```python
from build123d import *

# Parameters (mm, degrees)
F0_R     = 38.1
F1_DEPTH = 5.08


with BuildPart() as f1:
    # F0 (on Top) → F1 (new body)
    with BuildSketch(Plane.XY):
        Circle(F0_R)
        with BuildLine():
            ThreePointArc((21.9970452561, 12.7), (24.5345159877, 6.5740037456), (25.4, 0))
            ThreePointArc((25.4, 0), (24.5345159877, -6.5740037456), (21.9970452561, -12.7))
            ThreePointArc((21.9970452561, -12.7), (17.9605122421, -17.9605122421), (12.7, -21.9970452561))
            ThreePointArc((12.7, -21.9970452561), (6.5740037456, -24.5345159877), (0, -25.4))
            ThreePointArc((0, -25.4), (-6.5740037456, -24.5345159877), (-12.7, -21.9970452561))
            ThreePointArc((-12.7, -21.9970452561), (-17.9605122421, -17.9605122421), (-21.9970452561, -12.7))
            ThreePointArc((-21.9970452561, -12.7), (-24.5345159877, -6.5740037456), (-25.4, 0))
            ThreePointArc((-25.4, 0), (-24.5345159877, 6.5740037456), (-21.9970452561, 12.7))
            ThreePointArc((-21.9970452561, 12.7), (-17.9605122421, 17.9605122421), (-12.7, 21.9970452561))
            ThreePointArc((-12.7, 21.9970452561), (-6.5740037456, 24.5345159877), (0, 25.4))
            ThreePointArc((0, 25.4), (6.5740037456, 24.5345159877), (12.7, 21.9970452561))
            ThreePointArc((12.7, 21.9970452561), (17.9605122421, 17.9605122421), (21.9970452561, 12.7))
        make_face(mode=Mode.SUBTRACT)
        with BuildLine():
            Line((-8.248891971, -4.7625), (0, 0))
            Line((0, 0), (-9.525, 0))
            ThreePointArc((-9.525, 0), (-9.2004434954, -2.4652514046), (-8.248891971, -4.7625))
        make_face()
        with BuildLine():
            Line((-4.7625, -8.248891971), (0, 0))
            Line((0, 0), (-8.248891971, -4.7625))
            ThreePointArc((-8.248891971, -4.7625), (-6.7351920908, -6.7351920908), (-4.7625, -8.248891971))
        make_face()
        with BuildLine():
            Line((0, -9.525), (0, 0))
            Line((0, 0), (-4.7625, -8.248891971))
            ThreePointArc((-4.7625, -8.248891971), (-2.4652514046, -9.2004434954), (0, -9.525))
        make_face()
        with BuildLine():
            Line((4.7625, -8.248891971), (0, 0))
            Line((0, 0), (0, -9.525))
            ThreePointArc((0, -9.525), (2.4652514046, -9.2004434954), (4.7625, -8.248891971))
        make_face()
        with BuildLine():
            ThreePointArc((4.7625, -8.248891971), (6.7351920908, -6.7351920908), (8.248891971, -4.7625))
            Line((8.248891971, -4.7625), (0, 0))
            Line((0, 0), (4.7625, -8.248891971))
        make_face()
        with BuildLine():
            ThreePointArc((8.248891971, -4.7625), (9.2004434954, -2.4652514046), (9.525, 0))
            Line((9.525, 0), (0, 0))
            Line((0, 0), (8.248891971, -4.7625))
        make_face()
        with BuildLine():
            Line((0, 0), (9.525, 0))
            ThreePointArc((9.525, 0), (9.2004434954, 2.4652514046), (8.248891971, 4.7625))
            Line((8.248891971, 4.7625), (0, 0))
        make_face()
        with BuildLine():
            Line((0, 0), (8.248891971, 4.7625))
            ThreePointArc((8.248891971, 4.7625), (6.7351920908, 6.7351920908), (4.7625, 8.248891971))
            Line((4.7625, 8.248891971), (0, 0))
        make_face()
        with BuildLine():
            Line((0, 9.525), (0, 0))
            Line((0, 0), (4.7625, 8.248891971))
            ThreePointArc((4.7625, 8.248891971), (2.4652514046, 9.2004434954), (0, 9.525))
        make_face()
        with BuildLine():
            Line((-4.7625, 8.248891971), (0, 0))
            Line((0, 0), (0, 9.525))
            ThreePointArc((0, 9.525), (-2.4652514046, 9.2004434954), (-4.7625, 8.248891971))
        make_face()
        with BuildLine():
            Line((-8.248891971, 4.7625), (0, 0))
            Line((0, 0), (-4.7625, 8.248891971))
            ThreePointArc((-4.7625, 8.248891971), (-6.7351920908, 6.7351920908), (-8.248891971, 4.7625))
        make_face()
        with BuildLine():
            Line((-9.525, 0), (0, 0))
            Line((0, 0), (-8.248891971, 4.7625))
            ThreePointArc((-8.248891971, 4.7625), (-9.2004434954, 2.4652514046), (-9.525, 0))
        make_face()
        with BuildLine():
            ThreePointArc((-9.525, 0), (-9.2004434954, 2.4652514046), (-8.248891971, 4.7625))
            Line((-8.248891971, 4.7625), (-21.9970452561, 12.7))
            ThreePointArc((-21.9970452561, 12.7), (-24.5345159877, 6.5740037456), (-25.4, 0))
            Line((-25.4, 0), (-9.525, 0))
        make_face()
        with BuildLine():
            Line((0, 9.525), (0, 25.4))
            ThreePointArc((0, 25.4), (-6.5740037456, 24.5345159877), (-12.7, 21.9970452561))
            Line((-12.7, 21.9970452561), (-4.7625, 8.248891971))
            ThreePointArc((-4.7625, 8.248891971), (-2.4652514046, 9.2004434954), (0, 9.525))
        make_face()
        with BuildLine():
            Line((8.248891971, 4.7625), (21.9970452561, 12.7))
            ThreePointArc((21.9970452561, 12.7), (17.9605122421, 17.9605122421), (12.7, 21.9970452561))
            Line((12.7, 21.9970452561), (4.7625, 8.248891971))
            ThreePointArc((4.7625, 8.248891971), (6.7351920908, 6.7351920908), (8.248891971, 4.7625))
        make_face()
        with BuildLine():
            ThreePointArc((21.9970452561, -12.7), (24.5345159877, -6.5740037456), (25.4, 0))
            Line((25.4, 0), (9.525, 0))
            ThreePointArc((9.525, 0), (9.2004434954, -2.4652514046), (8.248891971, -4.7625))
            Line((8.248891971, -4.7625), (21.9970452561, -12.7))
        make_face()
        with BuildLine():
            ThreePointArc((0, -25.4), (6.5740037456, -24.5345159877), (12.7, -21.9970452561))
            Line((12.7, -21.9970452561), (4.7625, -8.248891971))
            ThreePointArc((4.7625, -8.248891971), (2.4652514046, -9.2004434954), (0, -9.525))
            Line((0, -9.525), (0, -25.4))
        make_face()
        with BuildLine():
            ThreePointArc((-4.7625, -8.248891971), (-6.7351920908, -6.7351920908), (-8.248891971, -4.7625))
            Line((-8.248891971, -4.7625), (-21.9970452561, -12.7))
            ThreePointArc((-21.9970452561, -12.7), (-17.9605122421, -17.9605122421), (-12.7, -21.9970452561))
            Line((-12.7, -21.9970452561), (-4.7625, -8.248891971))
        make_face()
    extrude(amount=F1_DEPTH)


solid = f1.part
```
Work out the finished part from the listing and answer in its coordinate system (mm). A direction names the side the tool comes from. Give positions to 0.01 mm unless a question says otherwise; leave off trailing zeros. Loops run counter-clockwise (first coordinate to the right, second up) from the corner with the lowest first, then second, coordinate; pieces in that order, holes last. Notation, with made-up numbers: (86, 3) - (93, 3) arc R28 ccw to (93, 32) - close; hole circle Ø8 at (-21.5, -32.5). An arc over 180 degrees is marked (long way). One line per question, with ' | ' between items.
(1) The part is cut by section B-B (x = 20.5). Write down the section's boundary in (y, z).
Recorded:
outline: (-32.11, 0) - (-15, 0) - (-15, 5.08) - (-32.11, 5.08) - close; (-11.84, 0) - (0, 0) - (0, 5.08) - (-11.84, 5.08) - close; (11.84, 0) - (32.11, 0) - (32.11, 5.08) - (11.84, 5.08) - close
(2) The part is cut by section C-C (z = 3.25). Count the separate pieces of the cut face and the enclosed holes in it, then the cut area to 3 significant figures.
Recorded:
separate pieces: 1 | enclosed holes: 6 | area: 3,690 mm²
(3) A tool of negligible diameter and unlimited length cuts with its end or side. For faces 1 (the face through (-1, 1, 5.08)), 2 (the face through (-15.027, -8.676, 2.504)), from which of +Z, -Z, +X, -X, +Y, -Y can it reach the whole face along a straight path? Write none if from no direction.
Recorded:
face 1: +Z, +X, -X, +Y, -Y | face 2: +Z, -Z
(4) Each of these flat-tipped pins is pushed along its axis until it touches: pin 1 Ø2 at (x, z) = (6, 2.5) entering from -Y; pin 2 Ø1 at (x, z) = (-8.5, 0.5) entering from -Y; pin 3 Ø3 at (x, z) = (-22, 1) entering from -Y. Where does it stop, or does it pass through?
Recorded:
pin 1: stops at y = -37.77 | pin 2: stops at y = -37.25 | pin 3: stops at y = -32.11
(5) The mould has two halves that part along Y. Classify faces 3 (the face through (-1, 1, 0)), 4 (the face through (-24.5, -6.7, 2.5)): +Y half, -Y half, draft (parallel to the pull), parting line (faces both ways), or undercut.
Recorded:
face 3: draft | face 4: undercut
(6) The part is cut by section D-D (y = -15). Write down the section's boundary in (x, z), then the cut area to 3 significant figures.
Recorded:
outline: (-35.02, 0) - (-8.66, 0) - (-8.66, 5.08) - (-35.02, 5.08) - close; (0, 0) - (8.66, 0) - (8.66, 5.08) - (0, 5.08) - close; (20.5, 0) - (35.02, 0) - (35.02, 5.08) - (20.5, 5.08) - close | area: 252 mm²
(7) Straight lines are drawn through the part: probe 1 along X at (y, z) = (-12, 1.7); probe 2 along Y at (x, z) = (14, 4.8); probe 3 along Y at (x, z) = (0.5, 3.55). For each, find the intervals that lie inside material, in ascending order.
Recorded:
probe 1: x = -36.16 to -22.39, -20.78 to -6.93, 0 to 6.93, 20.78 to 36.16 | probe 2: y = -35.43 to -21.19, -8.08 to 0, 8.08 to 35.43 | probe 3: y = -38.1 to 9.51, 25.4 to 38.1
(8) The part is cut by section A-A (y = 11). Write down the section's boundary in (x, z).
Recorded:
outline: (-36.48, 0) - (-19.05, 0) - (-19.05, 5.08) - (-36.48, 5.08) - close; (-6.35, 0) - (0, 0) - (0, 5.08) - (-6.35, 5.08) - close; (6.35, 0) - (19.05, 0) - (19.05, 5.08) - (6.35, 5.08) - close; (22.89, 0) - (36.48, 0) - (36.48, 5.08) - (22.89, 5.08) - close
